For this review, take the finished solid that the model builds, in its own axes (mm). A direction names the side the tool comes from. Coordinates: 2 decimals unless noted, no trailing zeros. Write each loop counter-clockwise with the first axis right and the second up, starting at its lowest first coordinate (ties: lowest second). Pieces come first, ordered by that corner, then holes. Notation, with made-up numbers: M 75,-19.5 L 114,-19.5 A27 cw 114,4.5 Z; hole C 46,13.25 d6. An arc over 180 degrees is marked long. Return JSON: item names as keys, results as strings.
```python
from build123d import *

# Parameters (mm, degrees)
SKETCH_1_W          = 71
SKETCH_1_H          = 18
EXTRUDE_1_DEPTH     = 13
SKETCH_2_R          = 1
SKETCH_2_R_2        = 2
CUT_EXTRUDE_1_DEPTH = 75.390859654
SKETCH_3_R          = 1.65
CUT_EXTRUDE_2_DEPTH = 75.390859654
CUT_EXTRUDE_3_DEPTH = 5
SKETCH_5_R          = 11.5
CUT_EXTRUDE_4_DEPTH = 3
SKETCH_6_R          = 3
CUT_EXTRUDE_5_DEPTH = 2


with BuildPart() as part:
    # Sketch 1 → Extrude 1 (new body)
    with BuildSketch(Plane.XY):
        with Locations((35.5, 9)):
            Rectangle(SKETCH_1_W, SKETCH_1_H)
    extrude(amount=EXTRUDE_1_DEPTH)

    # Sketch 2 → Cut-Extrude 1 (cut, through all)
    with BuildSketch(Plane(origin=(0, 0, 0), x_dir=(-1, 0, 0), z_dir=(0, 0, -1))):
        with Locations((-35.5, 8)):
            Circle(SKETCH_2_R)
        with Locations((-10.5, 8)):
            Circle(SKETCH_2_R_2)
        with Locations((-60.5, 8)):
            Circle(SKETCH_2_R_2)
    extrude(amount=-CUT_EXTRUDE_1_DEPTH, mode=Mode.SUBTRACT)

    # Sketch 3 → Cut-Extrude 2 (cut, through all)
    with BuildSketch(Plane(origin=(0, 18, 0), x_dir=(1, 0, 0), z_dir=(0, 1, 0))):
        with Locations(Location((57.15, -5.5, 0), (0, 0, 270))):
            Circle(SKETCH_3_R)
        with Locations(Location((26.15, -5.5, 0), (0, 0, 270))):
            Circle(SKETCH_3_R)
    extrude(amount=-CUT_EXTRUDE_2_DEPTH, mode=Mode.SUBTRACT)

    # Sketch 4 → Cut-Extrude 3 (cut)
    with BuildSketch(Plane.XY.offset(13)):
        Polygon((60.5, 11.464101615), (57.5, 9.732050808), (57.5, 6.267949192), (60.5, 4.535898385), (63.5, 6.267949192), (63.5, 9.732050808), align=None)
        Polygon((13.5, 9.732050808), (10.5, 11.464101615), (7.5, 9.732050808), (7.5, 6.267949192), (10.5, 4.535898385), (13.5, 6.267949192), align=None)
    extrude(amount=-CUT_EXTRUDE_3_DEPTH, mode=Mode.SUBTRACT)

    # Sketch 5 → Cut-Extrude 4 (cut)
    with BuildSketch(Plane(origin=(0, 18, 0), x_dir=(1, 0, 0), z_dir=(0, 1, 0))):
        with Locations((41.65, -21)):
            Circle(SKETCH_5_R)
    extrude(amount=-CUT_EXTRUDE_4_DEPTH, mode=Mode.SUBTRACT)

    # Sketch 6 → Cut-Extrude 5 (cut)
    with BuildSketch(Plane.XZ):
        with Locations(Location((26.15, 5.5, 0), (0, 0, 270))):
            Circle(SKETCH_6_R)
        with Locations(Location((57.15, 5.5, 0), (0, 0, 270))):
            Circle(SKETCH_6_R)
    extrude(amount=-CUT_EXTRUDE_5_DEPTH, mode=Mode.SUBTRACT)


solid = part.part
```
1. We need section A-A (z = 5.5). State the section outline as (x, y) points.
Checks:
{"outline": "M 0,0 L 23.15,0 L 23.15,2 L 24.5,2 L 24.5,18 L 0,18 Z; M 27.8,2 L 29.15,2 L 29.15,0 L 54.15,0 L 54.15,2 L 55.5,2 L 55.5,18 L 27.8,18 Z; M 58.8,2 L 60.15,2 L 60.15,0 L 71,0 L 71,18 L 58.8,18 L 58.8,9.05 A2 cw long 58.8,6.95 Z; hole C 10.5,8 d4; hole C 35.5,8 d2"}
2. Clearance check with flat-ended pins moving along their axes: pin 1 Ø1 at (y, z) = (7, 10) entering from -X; pin 2 Ø3 at (x, z) = (58.5, 6) entering from -Y; pin 3 Ø3 at (x, y) = (9.5, 8) entering from +Z; pin 4 Ø1 at (x, z) = (43.5, 11) entering from +Y. State where each tip first meets the part, or that it passes through.
Checks:
{"pin 1": "x = 0", "pin 2": "y = 2", "pin 3": "z = 8", "pin 4": "y = 15"}
3. We need section B-B (y = 16). State the section outline as (x, z) points, plus the area to 3 significant figures.
Checks:
{"outline": "M 0,0 L 71,0 L 71,13 L 49.91,13 A11.5 cw 33.39,13 L 0,13 Z; hole C 26.15,5.5 d3.3; hole C 57.15,5.5 d3.3", "area": "866 mm2"}
4. Wall thickness on L1, parallel to X at y = 11, z = 4.25; L2, parallel to X at y = 0.6, z = 5.5; L3, parallel to Y at x = 60.5, z = 4.5: over which ranges is each line inside the solid? List them lowest first. Write a range as from..to.
Checks:
{"L1": "0..25.07, 27.23..56.07, 58.23..71", "L2": "0..23.15, 29.15..54.15, 60.15..71", "L3": "0..6, 10..18"}
5. We need section C-C (y = 3.5). State the section outline as (x, z) points.
Checks:
{"outline": "M 0,0 L 71,0 L 71,13 L 0,13 Z; hole C 26.15,5.5 d3.3; hole C 57.15,5.5 d3.3"}
6. For faces 5 (the face through (42, 15, 12)), 6 (the face through (12, 5.4, 10.5)), 7 (the face through (62.498, 8.088, 3.944)), 8 (the face through (35, 9.1, 13)), 9 (the face through (56, 2, 4)), list the 3-axis set-ups (+Z, -Z, +X, -X, +Y, -Y) from which the entire face can be reached by the end or side of a thin tool; tool diameter is ignored.
Checks:
{"face 5": "+Z, +Y", "face 6": "+Z", "face 7": "+Z, -Z", "face 8": "+Z, +X, -X, +Y, -Y", "face 9": "-Y"}
7. Draft analysis for pull direction X (two halves, no side actions). For faces 1 (the face through (35, 18, 6)), 2 (the face through (13.5, 8, 11)), 3 (the face through (24.54, 10.11, 5.14)), 4 (the face through (71, 9, 6)), state which applies: +X half, -X half, draft (parallel to the pull), parting line (faces both ways), or undercut.
Checks:
{"face 1": "draft", "face 2": "undercut", "face 3": "undercut", "face 4": "+X half"}
